Build history of the part. All positions in model axes, mm. A direction names the side the tool comes from. Give positions to 0.01 mm unless a question says otherwise; leave off trailing zeros. Order: outer loops, then holes, each group sorted by start corner. A loop starts at its lowest first (then second) coordinate and runs counter-clockwise, first axis right, second up. Notation, with made-up numbers: M 62,-18.5 L 92,-18.5 A21 cw 92,0.5 Z; hole C -16,-4.75 d4. An arc over 180 degrees is marked long. One line per item, written item: value.
from build123d import *

# Parameters (mm, degrees)
EXTRUDE_1_DEPTH        = 15
CUT_EXTRUDE_1_DEPTH    = 14
SKETCH_7_W             = 46
SKETCH_7_H             = 6
CUT_EXTRUDE_2_DEPTH    = 1
SKETCH_8_W             = 14
SKETCH_8_H             = 4
CUT_EXTRUDE_3_DEPTH    = 1
CUT_EXTRUDE_6_DEPTH    = 1
EXTRUDE_START          = -30
EXTRUDE_10_OUTLINE_W   = 3
EXTRUDE_10_OUTLINE_H   = 17.5
EXTRUDE_10_OUTLINE_H_2 = 10.5
EXTRUDE_10_OUTLINE_W_2 = 9
EXTRUDE_10_OUTLINE_H_3 = 1
EXTRUDE_10_OUTLINE_W_3 = 2
EXTRUDE_10_DEPTH       = 30
SKETCH_29_W            = 29
SKETCH_29_H            = 25.5
EXTRUDE_12_DEPTH       = 1.5
SKETCH_30_R            = 2.2
SKETCH_30_W            = 9
SKETCH_30_H            = 9
CUT_EXTRUDE_8_DEPTH    = 1.5
SKETCH_31_W            = 1.75
SKETCH_31_H            = 1
EXTRUDE_13_DEPTH       = 15
SKETCH_33_W            = 9
SKETCH_33_H            = 1
SKETCH_33_W_2          = 3.75
CUT_EXTRUDE_9_DEPTH    = 15
SKETCH_38_W            = 3
SKETCH_38_H            = 10.5
CUT_EXTRUDE_11_DEPTH   = 15
SKETCH_39_W            = 29
SKETCH_39_H            = 1
EXTRUDE_14_DEPTH       = 30
SKETCH_40_W            = 48
SKETCH_40_H            = 8
CUT_EXTRUDE_12_DEPTH   = 15


# Read off the part's stored shape, not the designer's step: 凸台-拉伸10
with BuildPart() as part:
    # 草图3 → 凸台-拉伸1 (new body)
    with BuildSketch(Plane.XY):
        Polygon((-25, 21.5), (23, 21.5), (23, 13.5), (6.5, 13.5), (6.5, 8), (17.5, 8), (17.5, -1), (12.5, -1), (12.5, -17.5), (-12.5, -17.5), (-12.5, -1), (-17.5, -1), (-17.5, 8), (-11.75, 8), (-11.75, 13.5), (-25, 13.5), align=None)
    extrude(amount=EXTRUDE_1_DEPTH)

    # 草图4 → 切除-拉伸1 (cut)
    with BuildSketch(Plane.XY.offset(15)):
        Polygon((22, 20.5), (-24, 20.5), (-24, 14.5), (-10.75, 14.5), (-10.75, 7), (-16.5, 7), (-16.5, 0), (-11.5, 0), (-11.5, -16.5), (11.5, -16.5), (11.5, 0), (16.5, 0), (16.5, 7), (5.5, 7), (5.5, 14.5), (22, 14.5), align=None)
    extrude(amount=-CUT_EXTRUDE_1_DEPTH, mode=Mode.SUBTRACT)

    # 草图7 → 切除-拉伸2 (cut)
    with BuildSketch(Plane.XY.offset(1)):
        with Locations((-1, 17.5)):
            Rectangle(SKETCH_7_W, SKETCH_7_H)
    extrude(amount=-CUT_EXTRUDE_2_DEPTH, mode=Mode.SUBTRACT)

    # 草图8 → 切除-拉伸3 (cut)
    with BuildSketch(Plane.ZY.offset(12.5)):
        with Locations((8, -12.5)):
            Rectangle(SKETCH_8_W, SKETCH_8_H)
    extrude(amount=-CUT_EXTRUDE_3_DEPTH, mode=Mode.SUBTRACT)

    # 草图9 → 切除-拉伸6 (cut)
    with BuildSketch(Plane(origin=(0, 0, 0), x_dir=(-1, 0, 0), z_dir=(0, 0, -1))):
        Polygon((-3.5, 11.5), (-3.5, 5), (-14.5, 5), (-14.5, 2), (-9.5, 2), (-9.5, -14.5), (9.5, -14.5), (9.5, 2), (14.5, 2), (14.5, 5), (8.75, 5), (8.75, 11.5), align=None)
    extrude(amount=-CUT_EXTRUDE_6_DEPTH, mode=Mode.SUBTRACT)

    # 凸台-拉伸10 outline → 凸台-拉伸10 (add)
    with BuildSketch(Plane(origin=(0, 0, 0), x_dir=(-1, 0, 0), z_dir=(0, 0, -1)).offset(EXTRUDE_START)):
        with Locations((-13, -8.75)):
            Rectangle(EXTRUDE_10_OUTLINE_W, EXTRUDE_10_OUTLINE_H)
        Polygon((14.5, -15.5), (12.5, -14.5), (11.5, -14.5), (11.5, -17.5), (14.5, -17.5), align=None)
        with Locations((13, -5.25)):
            Rectangle(EXTRUDE_10_OUTLINE_W, EXTRUDE_10_OUTLINE_H_2)
        with Locations((-10, 7.5)):
            Rectangle(EXTRUDE_10_OUTLINE_W_2, EXTRUDE_10_OUTLINE_H_3)
        with Locations((13.5, 7.5)):
            Rectangle(EXTRUDE_10_OUTLINE_W_3, EXTRUDE_10_OUTLINE_H_3)
    extrude(amount=EXTRUDE_10_DEPTH)

    # 草图29 → 凸台-拉伸12 (add)
    with BuildSketch(Plane.XY.offset(30)):
        with Locations((0, -4.75)):
            Rectangle(SKETCH_29_W, SKETCH_29_H)
    extrude(amount=EXTRUDE_12_DEPTH)

    # 草图30 → 切除-拉伸8 (cut)
    with BuildSketch(Plane.XY.offset(31.5)):
        with Locations((-10, 1.25)):
            Circle(SKETCH_30_R)
        with Locations((-10, -10.75)):
            Circle(SKETCH_30_R)
        with Locations((10, 1.25)):
            Circle(SKETCH_30_R)
        with Locations((10, -10.75)):
            Circle(SKETCH_30_R)
        with Locations((0, -4.75)):
            Rectangle(SKETCH_30_W, SKETCH_30_H)
    extrude(amount=-CUT_EXTRUDE_8_DEPTH, mode=Mode.SUBTRACT)

    # 草图31 → 凸台-拉伸13 (add)
    with BuildSketch(Plane.XY.offset(15)):
        with Locations((-11.625, 7.5)):
            Rectangle(SKETCH_31_W, SKETCH_31_H)
    extrude(amount=EXTRUDE_13_DEPTH)

    # 草图33 → 切除-拉伸9 (cut)
    with BuildSketch(Plane.XY.offset(15)):
        with Locations((10, 7.5)):
            Rectangle(SKETCH_33_W, SKETCH_33_H)
        with Locations((-12.625, 7.5)):
            Rectangle(SKETCH_33_W_2, SKETCH_33_H)
    extrude(amount=CUT_EXTRUDE_9_DEPTH, mode=Mode.SUBTRACT)

    # 草图38 → 切除-拉伸11 (cut)
    with BuildSketch(Plane.XY.offset(15)):
        with Locations((-13, -5.25)):
            Rectangle(SKETCH_38_W, SKETCH_38_H)
    extrude(amount=CUT_EXTRUDE_11_DEPTH, mode=Mode.SUBTRACT)

    # 草图39 → 凸台-拉伸14 (add)
    with BuildSketch(Plane(origin=(0, 0, 0), x_dir=(-1, 0, 0), z_dir=(0, 0, -1))):
        with Locations((0, -17)):
            Rectangle(SKETCH_39_W, SKETCH_39_H)
    extrude(amount=-EXTRUDE_14_DEPTH)

    # 草图40 → 切除-拉伸12 (cut)
    with BuildSketch(Plane(origin=(0, 0, 0), x_dir=(-1, 0, 0), z_dir=(0, 0, -1))):
        with Locations((1, 17.5)):
            Rectangle(SKETCH_40_W, SKETCH_40_H)
    extrude(amount=-CUT_EXTRUDE_12_DEPTH, mode=Mode.SUBTRACT)


solid = part.part
1) Pin check, flat tips, straight feed: pin 1 (8 mm diameter, centred on y = -4, z = 20.5, fed in from +X); pin 2 (5 mm diameter, centred on y = -7.5, z = 4.5, fed in from -X); pin 3 (0.9 mm diameter, centred on x = 16.5, z = 9.5, fed in from -Y). Stop position of each tip, or through.
Check values:
pin 1: x = 14.5
pin 2: x = -14.5
pin 3: y = -1
2) Saw through at D-D, the plane y = 1.25. Write the cut outline in (x, z), then the cut area to 3 significant figures.
Check values:
outline: M -17.5,0 L -9.5,0 L -9.5,1 L -16.5,1 L -16.5,15 L -17.5,15 Z; M -14.5,30 L -12.2,30 L -12.2,31.5 L -14.5,31.5 Z; M -7.8,30 L 7.8,30 L 7.8,31.5 L -7.8,31.5 Z; M 9.5,0 L 17.5,0 L 17.5,15 L 16.5,15 L 16.5,1 L 9.5,1 Z; M 12.2,30 L 14.5,30 L 14.5,31.5 L 12.2,31.5 Z
area: 74.3 mm^2
3) Drill centre lines: probe 1 along Y at (x, z) = (10, 30.7); probe 2 along Y at (x, z) = (-12.5, 5.5); probe 3 along Z at (x, y) = (11, -8.5). Where is each one in solid material? Low to high. Write a range as from..to.
Check values:
probe 1: -17.5..-12.95, -8.55..-0.95, 3.45..8
probe 2: -17.5..-14.5, -10.5..0, 7..8
probe 3: 0..1, 30..31.5
4) Saw through at A-A, the plane y = -8. Write the cut outline in (x, z).
Check values:
outline: M -14.5,0 L -9.5,0 L -9.5,1 L -11.5,1 L -11.5,15 L -14.5,15 Z; M -14.5,30 L -4.5,30 L -4.5,31.5 L -14.5,31.5 Z; M 4.5,30 L 11.5,30 L 11.5,1 L 9.5,1 L 9.5,0 L 14.5,0 L 14.5,31.5 L 4.5,31.5 Z
5) Mould opens along Z. For faces 6 (the face through (-14, -1, 15)), 7 (the face through (-14.5, -16, 20)) say: released by +Z, released by -Z, zero draft, split by the parting line, or undercut.
Check values:
face 6: undercut
face 7: zero draft
6) Tool access for faces 1 (the face through (-4.5, -5, 31)), 2 (the face through (11.5, -8, 16)), 3 (the face through (-13, -10.5, 7)), 4 (the face through (8.38, -9.26, 30.76)), 5 (the face through (-11.75, 11, 7)): list every direction of +Z, -Z, +X, -X, +Y, -Y with a clear straight run to the whole face (end or side of a thin tool).
Check values:
face 1: +Z, -Z
face 2: none
face 3: -X
face 4: +Z
face 5: +Z, -Z, -X, +Y
7) Saw through at B-B, the plane x = -10. Write the cut outline in (y, z), then the cut area to 4 significant figures.
Check values:
outline: M -17.5,0 L 2,0 L 2,1 L -16.5,1 L -16.5,30 L -12.95,30 L -12.95,31.5 L -17.5,31.5 Z; M -8.55,30 L -0.95,30 L -0.95,31.5 L -8.55,31.5 Z; M 3.45,30 L 8,30 L 8,31.5 L 3.45,31.5 Z; M 5,0 L 13.5,0 L 13.5,1 L 5,1 Z
area: 82.05 mm^2
